Geometry: final body of the model. Coordinates: model frame, mm. Face numbers are marked on the shaded views. A direction names the side the tool comes from. Round coordinates to 2 decimals unless told otherwise and drop trailing zeros. Write each loop counter-clockwise with the first axis right and the second up, starting at its lowest first coordinate (ties: lowest second). Pieces come first, ordered by that corner, then holes. Notation, with made-up numbers: M 45.5,11.5 L 86.5,11.5 A31 cw 86.5,38.5 Z; hole C 2,38 d4. An arc over 180 degrees is marked long. Use one line per item in the form item = value. Start each with the question number.
Item 1: Section query D-D (y = 41.5). Return loops of the section in (x, z), and give its area (3 significant figures).
Item 2: Section query B-B (y = 32.5). Return loops of the section in (x, z), and give its area (3 significant figures).
Item 3: Ray query, probe 1 along X at (y, z) = (24, 17); probe 2 along Y at (x, z) = (64.5, 8.5); probe 3 along Z at (x, y) = (5.3, 32.5). Return the intervals inside material, ascending.
Item 4: Section query A-A (z = 16). Return loops of the section in (x, y).
Item 5: Section query C-C (x = 49.5). Return loops of the section in (y, z).
Item 6: Reachability of the marked faces 5 and 6 from +Z, -Z, +X, -X, +Y, -Y: full face, straight path, thin tool, end or side. Return the list, or none.
Item 7: Pin query (flat end, axial travel): pin 1 Ø10 at (y, z) = (32.5, 8.81) entering from -X; pin 2 Ø1.5 at (x, y) = (100.5, 40) entering from +Z. Return the tip coordinate at first contact, or that it passes through.
Item 8: Pull-direction query (Y, two-part tool) for the marked faces 1, 2, 3 and 4; classes: pulls with the +Y half, pulls with the -Y half, needs draft (parallel to the pull), parting line crosses it, or undercut.
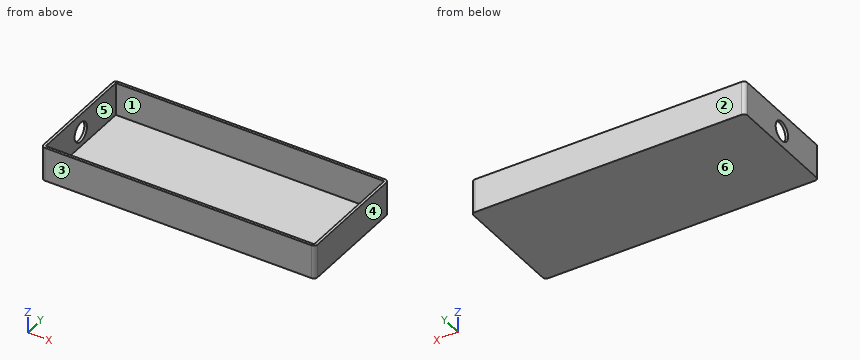
Autodesk Fusion 360 part; units mm, degrees
sketch "Sketch3" plane through (0, 0, 0) normal (0, 0, 1) x (1, 0, 0)
  line L0 (7, 0) -> (157.5, 0)
  line L1 (159.5, 2) -> (159.5, 63)
  line L2 (157.5, 65) -> (7, 65)
  line L3 (5, 63) -> (5, 2)
  arc A0 (7, 65) -> (5, 63) centre (7, 63) ccw
  arc A1 (159.5, 63) -> (157.5, 65) centre (157.5, 63) ccw
  arc A2 (157.5, 0) -> (159.5, 2) centre (157.5, 2) ccw
  arc A3 (5, 2) -> (7, 0) centre (7, 2) ccw
  dimension "d12" = 65
  dimension "d13" = 2
  dimension "d14" = 2
  dimension "d15" = 2
  dimension "d16" = 2
  dimension "d30" = 150.5
extrude "Extrude2" add sketch "Sketch3" along normal blind 12.7
extrude "Extrude3" add 1 faces at (107.3333, 21.6667, 12.7) along direction (0, 0, 1) blind 6.35
sketch "Sketch5" plane through (0, 0, 19.05) normal (0, 0, 1) x (-1, 0, 0)
  arc A0 (-5, -2) -> (-7, 0) centre (-7, -2) ccw
  line L0 (-7, 0) -> (-157.5, 0)
  arc A1 (-157.5, 0) -> (-159.5, -2) centre (-157.5, -2) ccw
  line L1 (-159.5, -2) -> (-159.5, -63)
  arc A2 (-159.5, -63) -> (-157.5, -65) centre (-157.5, -63) ccw
  line L2 (-157.5, -65) -> (-7, -65)
  arc A3 (-7, -65) -> (-5, -63) centre (-7, -63) ccw
  line L3 (-5, -63) -> (-5, -2)
  line L4 (-6.5, -63.5) -> (-158, -63.5)
  line L5 (-158, -63.5) -> (-158, -1.5)
  line L6 (-158, -1.5) -> (-6.5, -1.5)
  line L7 (-6.5, -1.5) -> (-6.5, -63.5)
  line L8 (-158, -1.5) -> (-158, -63.5)
  dimension "d26" = 1.5
  dimension "d27" = 1.5
  dimension "d28" = 1.5
  dimension "d29" = 1.5
extrude "Extrude4" cut sketch "Sketch5" against normal blind 10 contours L4 L5 L6 L7 L8
sketch "Sketch6" plane through (5, 0, 0) normal (-1, 0, 0) x (0, -1, 0)
  line L0 (-63, 0) -> (-2, 0)
  line L1 (-2, 0) -> (-2, 19.05)
  line L2 (-2, 19.05) -> (-63, 19.05)
  line L3 (-63, 19.05) -> (-63, 0)
  circle A0 centre (-32.5, 8.8069) radius 5.5
  dimension "d33" = 11
  dimension "d34" = 30.5
extrude "Extrude5" cut 1 faces at (57, 42.8333, 9.05) along direction (0, 0, -1) blind 5.35
extrude "Extrude6" cut 1 faces at (57, 42.8333, 3.7) along direction (0, 0, -1) blind 3.15
extrude "Extrude7" cut sketch "Sketch6" against normal blind 5 contours A0
Working result:
q1.outline = M 5,0 L 159.5,0 L 159.5,19.05 L 158,19.05 L 158,0.55 L 6.5,0.55 L 6.5,19.05 L 5,19.05 Z
q1.area = 140 mm²
q2.outline = M 5,0 L 159.5,0 L 159.5,19.05 L 158,19.05 L 158,0.55 L 6.5,0.55 L 6.5,3.31 L 5,3.31 Z; M 5,14.31 L 6.5,14.31 L 6.5,19.05 L 5,19.05 Z
q2.area = 124 mm²
q3.probe_1 = 5 to 6.5, 158 to 159.5
q3.probe_2 = 0 to 1.5, 63.5 to 65
q3.probe_3 = 0 to 3.31, 14.31 to 19.05
q4.outline = M 5,2 A2 ccw 7,0 L 157.5,0 A2 ccw 159.5,2 L 159.5,63 A2 ccw 157.5,65 L 7,65 A2 ccw 5,63 Z; hole M 6.5,1.5 L 158,1.5 L 158,63.5 L 6.5,63.5 Z
q5.outline = M 0,0 L 65,0 L 65,19.05 L 63.5,19.05 L 63.5,0.55 L 1.5,0.55 L 1.5,19.05 L 0,19.05 Z
q6.face_5 = +Z
q6.face_6 = -Z, +X, -X, +Y, -Y
q7.pin_1 = 158
q7.pin_2 = 0.55
q8.face_1 = undercut
q8.face_2 = pulls with the +Y half
q8.face_3 = pulls with the -Y half
q8.face_4 = needs draft
